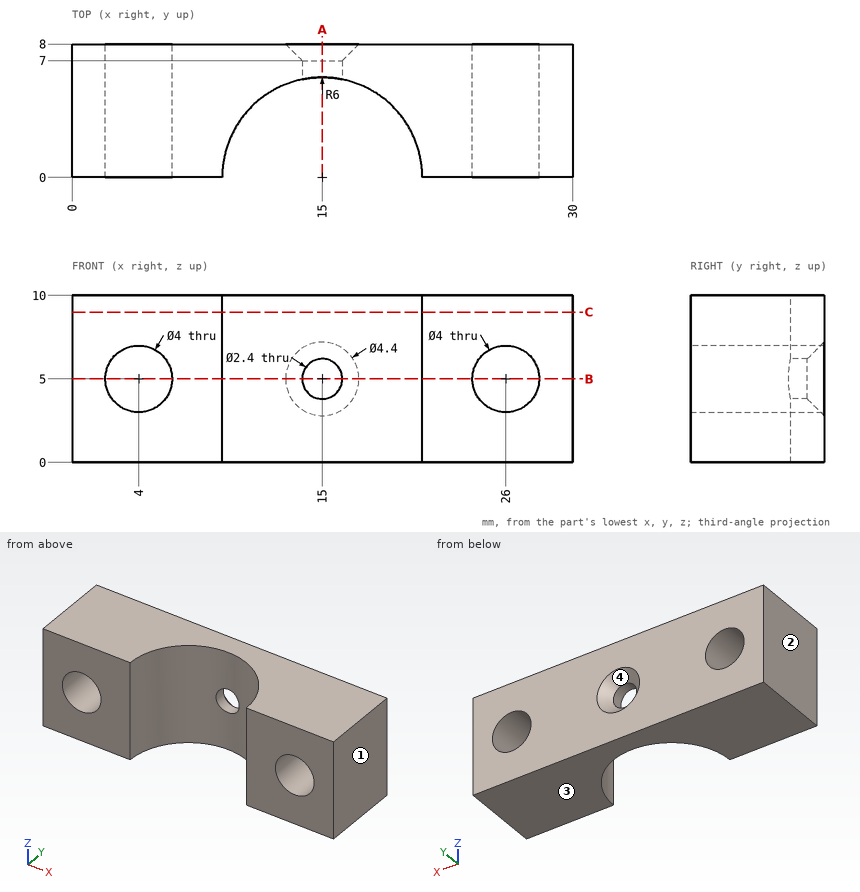
Check sheet for the drawn part. Datum: minimum x, y, z corner. Units: mm. Round coordinates to 2 decimals unless told otherwise and drop trailing zeros. Order: outer loops, then holes, each group sorted by start corner. A loop starts at its lowest first (then second) coordinate and runs counter-clockwise, first axis right, second up. Notation, with made-up numbers: (88.5, 27.5) -> (125.5, 27.5) arc R7 ccw to (125.5, 35.5) -> close; hole circle Ø5 at (52.5, 15). An arc over 180 degrees is marked (long way). Put each result on its own line as item: value. Start each with the question number.
(1) Section check C-C (z = 9). Enter the section's corners in (x, y), then the cut area to 3 significant figures.
(2) Material ranges on line 1 along X through (y, z) = (4.75, 5); line 2 along Z through (x, y) = (15, 6.55); line 3 along X through (y, z) = (4, 3.25), recorded low to high.
(3) Draft check along X on the marked faces 1, 2, 3 and 4. Enter one of: +X half, -X half, draft (parallel to the pull), parting line (faces both ways), or undercut.
(4) Section check B-B (z = 5). Enter the section's corners in (x, y), then the cut area to 3 significant figures.
(5) Depth check by flat-ended pin: pin 1 Ø4 at (x, z) = (15, 5) entering from -Y. Enter the tip coordinate at first touch or a pass-through.
(6) Section check A-A (x = 15). Enter the section's corners in (y, z), then the cut area to 3 significant figures.
Completed:
1. outline: (0, 0) -> (9, 0) arc R6 cw to (21, 0) -> (30, 0) -> (30, 8) -> (0, 8) -> close
1. area: 183 mm2
2. line 1: x = 0 to 2, 6 to 11.33, 18.67 to 24, 28 to 30
2. line 2: z = 0 to 3.8, 6.2 to 10
2. line 3: x = 0 to 3.03, 4.97 to 10.53, 19.47 to 25.03, 26.97 to 30
3. face 1: +X half
3. face 2: -X half
3. face 3: draft
3. face 4: undercut
4. outline: (0, 0) -> (2, 0) -> (2, 8) -> (0, 8) -> close; (6, 0) -> (9, 0) arc R6 cw to (13.8, 5.88) -> (13.8, 7) -> (12.8, 8) -> (6, 8) -> close; (16.2, 5.88) arc R6 cw to (21, 0) -> (24, 0) -> (24, 8) -> (17.2, 8) -> (16.2, 7) -> close; (28, 0) -> (30, 0) -> (30, 8) -> (28, 8) -> close
4. area: 114 mm2
5. pin 1: stops at y = 5.66
6. outline: (6, 0) -> (8, 0) -> (8, 2.8) -> (7, 3.8) -> (6, 3.8) -> close; (6, 6.2) -> (7, 6.2) -> (8, 7.2) -> (8, 10) -> (6, 10) -> close
6. area: 14.2 mm2
